Autodesk Inventor part; units mm, degrees
ref_plane "YZ Plane" through (0, 0, 0) normal (1, 0, 0) x (0, 1, 0)
ref_plane "XZ Plane" through (0, 0, 0) normal (0, 1, 0) x (-1, 0, 0)
ref_plane "XY Plane" through (0, 0, 0) normal (0, 0, 1) x (1, 0, 0)
sketch "Esquisse2" plane through (0, 0, 0) normal (0, 0, 1) x (1, 0, 0)
  line L0 (0, 0) -> (15, 0)
  line L1 (18, 3) -> (18, 33)
  line L2 (15, 36) -> (0, 36)
  line L3 (-3, 33) -> (-3, 3)
  line L4 (-3, 3) -> (0, 0)
  line L5 (0, 36) -> (-3, 33)
  line L6 (15, 36) -> (18, 33)
  line L7 (18, 3) -> (15, 0)
  line L8 (0, 36) -> (0, 0) construction
  line L9 (15, 0) -> (15, 36) construction
  line L10 (18, 33) -> (-3, 33) construction
  line L11 (18, 3) -> (-3, 3) construction
  dimension "d12" = 15
  dimension "d14" = 21
  dimension "d15" = 36
extrude "Extrusion1" add sketch "Esquisse2" along normal blind 24
sketch "Esquisse3" plane through (-3, 3, 0) normal (-1, 0, 0) x (0, 0, 1)
  line L0 (0, 0) -> (0, 30) construction
  line L1 (24, 30) -> (24, 0) construction
  line L2 (0, -3) -> (24, -3) construction
  line L3 (3, -3) -> (21, -3)
  line L4 (21, -3) -> (21, 2.6)
  line L5 (21, 2.6) -> (3, 2.6)
  line L6 (3, 2.6) -> (3, -3)
  line L7 (3, 2.6) -> (0, 2.6) construction
  line L8 (21, 2.6) -> (24, 2.6) construction
  dimension "d24" = 3
  dimension "d25" = 5.6
extrude "Extrusion2" cut sketch "Esquisse3" against normal through all
sketch "Esquisse4" plane through (0, 0, 0) normal (0, 0, -1) x (-1, 0, 0)
  line L0 (-15, 0) -> (0, 0) construction
  line L1 (0, 0) -> (3, 3) construction
  line L2 (0, 36) -> (-15, 36) construction
  circle A0 centre (-7.5, 3) radius 2.5
  line L3 (-15, 0) -> (-7.5, 3) construction
  line L4 (0, 0) -> (-7.5, 3) construction
  line L5 (-7.5, 3) -> (3, 3) construction
  circle A1 centre (-1.5, 3) radius 2.5
  circle A2 centre (-13.5, 3) radius 2.5
  circle A3 centre (-7.5, 3) radius 2.5
  dimension "d28" = 0.5
  dimension "d29" = 5
  dimension "d32" = 6
  dimension "d35" = 6
extrude "Extrusion3" cut sketch "Esquisse4" against normal through all
sketch "Esquisse5" plane through (0, 0, 0) normal (0, 0, -1) x (-1, 0, 0)
  circle A0 centre (-7.5, 3) radius 2.5 construction
  line L0 (3, 3) -> (3, 33) construction
  line L1 (0, 36) -> (-15, 36) construction
  line L2 (-7.5, 3) -> (-7.5, 36) construction
  circle A1 centre (-7.5, 27) radius 2.5
  line L3 (-7.5, 27) -> (3, 27) construction
  circle A2 centre (-1.5, 27) radius 2.5
  circle A3 centre (-13.5, 27) radius 2.5
  circle A4 centre (-7.5, 27) radius 2.5
  dimension "d40" = 5
  dimension "d41" = 24
  dimension "d44" = 6
  dimension "d47" = 6
extrude "Extrusion4" cut sketch "Esquisse5" against normal blind 3
sketch "Esquisse7" plane through (7.5, 27, 3) normal (0, 0, -1) x (-1, 0, 0)
  circle A0 centre (0, 0) radius 2.5
  circle A1 centre (0, 0) radius 2
  point P0 (7.5, -27)
  dimension "d54" = 4
extrude "Extrusion6" cut sketch "Esquisse7" against normal through all contours A1
sketch "Esquisse8" plane through (18, 3, 0) normal (1, 0, 0) x (0, 0, -1)
  line L0 (0, 30) -> (0, 0) construction
  line L1 (0, 26.5) -> (0, 21.5)
  line L2 (-24, 21.4697) -> (-24, 26.4697)
  line L3 (-24, 23.9697) -> (0, 24) construction
  line L4 (-21, 20.7349) -> (-3, 20.7349)
  line L5 (-3, 20.7349) -> (-3, 27.2349)
  line L6 (-3, 27.2349) -> (-21, 27.2349)
  line L7 (-21, 27.2349) -> (-21, 20.7349)
  line L8 (-21, 20.7349) -> (-3, 27.2349) construction
  line L9 (-3, 20.7349) -> (-21, 27.2349) construction
  line L10 (-21, 2.6) -> (-3, 2.6)
  line L11 (-12, 23.9849) -> (-12, 2.6) construction
  line L12 (-21, 2.7349) -> (-3, 2.7349)
  line L13 (-3, 2.7349) -> (-3, 9.2349)
  line L14 (-3, 9.2349) -> (-21, 9.2349)
  line L15 (-21, 9.2349) -> (-21, 2.7349)
  point P0 (0, -3)
  dimension "d57" = 6.5
  dimension "d58" = 18
  dimension "d74" = 18
extrude "Extrusion7" add sketch "Esquisse8" along normal blind 1.5
sketch "Esquisse9" plane through (19.5, 3, 0) normal (1, 0, 0) x (0, 0, -1)
  line L0 (-3, 20.7349) -> (-3, 27.2349) construction
  line L1 (-21, 27.2349) -> (-21, 20.7349) construction
  line L2 (-21, 23.9849) -> (-3, 23.9849) construction
  circle A0 centre (-12, 23.9849) radius 2.5
  line L3 (-15, 23.9849) -> (3, 23.9849) construction
  circle A1 centre (-6, 23.9849) radius 2.5
  line L4 (-27, 23.9849) -> (-9, 23.9849) construction
  circle A2 centre (-18, 23.9849) radius 2.5
  line L5 (-21, 23.9849) -> (-3, 23.9849) construction
  circle A3 centre (-12, 23.9849) radius 2.5
  line L6 (-21, 20.7349) -> (-3, 20.7349)
  line L7 (-12, 23.9849) -> (-12, 11.4292) construction
  circle A4 centre (-12, 5.9849) radius 2.5
  circle A5 centre (-6, 5.9849) radius 2.5
  circle A6 centre (-18, 5.9849) radius 2.5
  point P0 (0, -3)
  dimension "d61" = 5
  dimension "d64" = 6
  dimension "d67" = 6
  dimension "d81" = 18
extrude "Extrusion8" cut sketch "Esquisse9" against normal blind 3
sketch "Esquisse10" plane through (-3, 3, 0) normal (-1, 0, 0) x (0, 0, 1)
  line L0 (3, 27.2349) -> (21, 27.2349)
  line L1 (21, 27.2349) -> (21, 20.7349)
  line L2 (21, 20.7349) -> (3, 20.7349)
  line L3 (3, 20.7349) -> (3, 27.2349)
  line L4 (21, 9.2349) -> (21, 2.7349)
  line L5 (21, 2.7349) -> (3, 2.7349)
  line L6 (3, 2.7349) -> (3, 9.2349)
  line L7 (3, 9.2349) -> (21, 9.2349)
  point P0 (0, -3)
extrude "Extrusion9" add sketch "Esquisse10" along normal blind 1.5
sketch "Esquisse11" plane through (-4.5, 3, 0) normal (-1, 0, 0) x (0, 0, 1)
  circle A0 centre (6, 23.9849) radius 2.5
  circle A1 centre (12, 23.9849) radius 2.5
  circle A2 centre (18, 23.9849) radius 2.5
  circle A3 centre (18, 5.9849) radius 2.5
  circle A4 centre (12, 5.9849) radius 2.5
  circle A5 centre (6, 5.9849) radius 2.5
  point P0 (0, -3)
extrude "Extrusion10" cut sketch "Esquisse11" against normal blind 1.5
sketch "Esquisse12" plane through (-3, 3, 0) normal (-1, 0, 0) x (0, 0, 1)
  line L0 (21, 27.2349) -> (21, 20.7349)
  line L1 (21, 20.7349) -> (3, 20.7349)
  line L2 (3, 20.7349) -> (3, 27.2349)
  line L3 (3, 27.2349) -> (21, 27.2349)
  line L4 (21, 2.7349) -> (3, 2.7349)
  line L5 (3, 2.7349) -> (3, 9.2349)
  line L6 (3, 9.2349) -> (21, 9.2349)
  line L7 (21, 9.2349) -> (21, 2.7349)
  line L8 (21, 2.6) -> (21, 0)
  line L9 (21, 0) -> (24, 0)
  line L10 (24, 30) -> (24, 0)
  line L11 (0, 30) -> (24, 30)
  line L12 (0, 0) -> (0, 30)
  line L13 (0, 0) -> (3, 0)
  line L14 (3, 0) -> (3, 2.6)
  line L15 (3, 2.6) -> (21, 2.6)
  point P0 (0, -3)
sketch "Esquisse13" plane through (18, 3, 0) normal (1, 0, 0) x (0, 0, -1)
  line L0 (-21, 9.2349) -> (-3, 9.2349)
  line L1 (-3, 20.7349) -> (-18.5, 20.7349)
  line L2 (-18.5, 20.7349) -> (-18.5, 9.2349)
  line L3 (-18.5, 9.2349) -> (-3, 9.2349)
  line L4 (-3, 9.2349) -> (-3, 20.7349)
  point P0 (0, -3)
  dimension "d90" = 15.5
extrude "Extrusion11" cut sketch "Esquisse13" against normal blind 3
sketch "Esquisse14" plane through (18, 3, 0) normal (1, 0, 0) x (0, 0, -1)
  line L0 (-21, 20.7349) -> (-3, 20.7349)
  line L1 (-3, 9.2349) -> (-21, 9.2349)
  line L2 (-3, 20.7349) -> (-9, 20.7349)
  line L3 (-9, 20.7349) -> (-9, 9.2349)
  line L4 (-9, 9.2349) -> (-3, 9.2349)
  line L5 (-3, 9.2349) -> (-3, 20.7349)
  point P0 (0, -3)
  dimension "d93" = 6
extrude "Extrusion12" add sketch "Esquisse14" against normal blind 0.2
sketch "Esquisse16" plane through (-3, 3, 0) normal (-1, 0, 0) x (0, 0, 1)
  line L0 (3, 9.2349) -> (21, 9.2349) construction
  line L1 (3, 20.7349) -> (18.5, 20.7349)
  line L2 (18.5, 20.7349) -> (18.5, 9.2349)
  line L3 (18.5, 9.2349) -> (3, 9.2349)
  line L4 (3, 9.2349) -> (3, 20.7349)
  point P0 (0, -3)
  dimension "d96" = 15.5
extrude "Extrusion13" cut sketch "Esquisse16" against normal blind 3
sketch "Esquisse17" plane through (-3, 3, 0) normal (-1, 0, 0) x (0, 0, 1)
  line L0 (3, 20.7349) -> (9, 20.7349)
  line L1 (9, 20.7349) -> (9, 9.2197)
  line L2 (9, 9.2197) -> (3, 9.2197)
  line L3 (3, 9.2197) -> (3, 20.7349)
  line L4 (3, 9.2349) -> (3, 20.7349)
  point P0 (0, -3)
  dimension "d99" = 6
extrude "Extrusion14" add sketch "Esquisse17" against normal blind 0.2
fillet "Congé1" radius 1 9 edges at (18, 33, 12) (15, 36, 12) (0, 36, 12) (0, 0, 1.5) (0, 0, 22.5) (15, 0, 1.5) (18, 3, 1.5) (15, 0, 22.5) (18, 3, 22.5)
chamfer "Chanfrein1" distance 0.5 angle 45 2 edges at (-3, 17.9849, 18.5) (18, 17.9849, 18.5)
sketch "Esquisse18" plane through (0, 0, 24) normal (0, 0, 1) x (1, 0, 0)
  circle A0 centre (7.5, 27) radius 2
  circle A1 centre (1.5, 3) radius 2.5
  circle A2 centre (7.5, 3) radius 2.5
  circle A3 centre (13.5, 3) radius 2.5
  arc A4 (17.7071, 2.7071) -> (18, 3.4142) centre (17, 3.4142) ccw
  line L0 (18, 3.4142) -> (18, 32.5858)
  arc A5 (18, 32.5858) -> (17.7071, 33.2929) centre (17, 32.5858) ccw
  line L1 (17.7071, 33.2929) -> (15.2929, 35.7071)
  arc A6 (15.2929, 35.7071) -> (14.5858, 36) centre (14.5858, 35) ccw
  line L2 (14.5858, 36) -> (0.4142, 36)
  arc A7 (0.4142, 36) -> (-0.2929, 35.7071) centre (0.4142, 35) ccw
  line L3 (-0.2929, 35.7071) -> (-3, 33)
  line L4 (-3, 33) -> (-3, 3)
  line L5 (-3, 3) -> (-0.2929, 0.2929)
  arc A8 (-0.2929, 0.2929) -> (0.4142, 0) centre (0.4142, 1) ccw
  line L6 (0.4142, 0) -> (14.5858, 0)
  arc A9 (14.5858, 0) -> (15.2929, 0.2929) centre (14.5858, 1) ccw
  line L7 (15.2929, 0.2929) -> (17.7071, 2.7071)
  line L8 (19.5, 11.4849) -> (19.5, 6.4849)
  line L9 (19.5, 8.9849) -> (4.268, 8.9849) construction
  point P0 (0, 0)
properties part number "Motor"
Build history of the part. All positions in model axes, mm. A direction names the side the tool comes from. Coordinates: 2 decimals unless noted, no trailing zeros. Order: outer loops, then holes, each group sorted by start corner. A loop starts at its lowest first (then second) coordinate and runs counter-clockwise, first axis right, second up. Notation, with made-up numbers: (-28, 0.5) -> (7, 0.5) arc R29 cw to (7, 37.5) -> close; hole circle Ø4 at (-5.75, 44). An arc over 180 degrees is marked (long way). Answer in a Markdown table with one row per item. Add a question column.
Q1. Band-saw the part on D-D, the plane y = 4. Give the number of separate pieces and of enclosed holes in the cut face, then the cut area to 3 significant figures.
Q2. Band-saw the part on A-A, the plane x = 1.5. List the corners of the cut face in (y, z), then the cut area to 3 significant figures.
Q3. Band-saw the part on C-C, the plane x = 7.5. List the corners of the cut face in (y, z), then the cut area to 3 significant figures.
Q4. Mould opens along Y. For faces 1 (the face through (-4, 27, 3)), 2 (the face through (-1, 18, 3)), 3 (the face through (7, 0, 22)) say: +Y half, -Y half, draft (parallel to the pull), parting line (faces both ways), or undercut.
Q5. Which spindle directions (+Z, -Z, +X, -X, +Y, -Y) get a long thin tool onto all of the face, cutting with end or side? Do faces 4 (the face through (-3.76, 28.675, 16.157)), 5 (the face through (16.5, 27, 12)), 6 (the face through (19, 9, 21)), 7 (the face through (17.8, 18, 6)). Say none if no direction does.
Q6. Drop flat-ended pins along their axis: pin 1 (5.5 mm diameter, centred on y = 26, z = 19, fed in from +X); pin 2 (2 mm diameter, centred on x = 17, z = 10, fed in from -Y); pin 3 (3.5 mm diameter, centred on x = -3, z = 13, fed in from +Y); pin 4 (1.2 mm diameter, centred on x = -4, y = 8.5, fed in from +Z). Give the stop position or say it passes through.
Q7. Band-saw the part on B-B, the plane z = 22. List the corners of the cut face in (x, y).
Q8. Wall check: line 1 along Y through (x, z) = (-3.65, 12); line 2 along Z through (x, y) = (18.75, 9); line 3 along Y through (x, z) = (7.5, 1.15). Give the ranges that are in metal, low to high. Write a range as [from, to].
Answers follow:
| question | item | result |
|---|---|---|
| 1 | separate pieces | 8 |
| 1 | enclosed holes | 0 |
| 1 | area | 43.5 mm^2 |
| 2 | outline | (0, 0) -> (0.5, 0) -> (0.5, 3) -> (0, 3) -> close; (0, 21) -> (0.5, 21) -> (0.5, 24) -> (0, 24) -> close; (5.5, 0) -> (24.5, 0) -> (24.5, 3) -> (29.5, 3) -> (29.5, 0) -> (36, 0) -> (36, 24) -> (5.5, 24) -> (5.5, 21) -> (5.6, 21) -> (5.6, 3) -> (5.5, 3) -> close |
| 2 | area | 718 mm^2 |
| 3 | outline | (0, 0) -> (0.5, 0) -> (0.5, 3) -> (0, 3) -> close; (0, 21) -> (0.5, 21) -> (0.5, 24) -> (0, 24) -> close; (5.5, 0) -> (24.5, 0) -> (24.5, 3) -> (25, 3) -> (25, 24) -> (5.5, 24) -> (5.5, 21) -> (5.6, 21) -> (5.6, 3) -> (5.5, 3) -> close; (29, 3) -> (29.5, 3) -> (29.5, 0) -> (36, 0) -> (36, 24) -> (29, 24) -> close |
| 3 | area | 634 mm^2 |
| 4 | face 1 | draft |
| 4 | face 2 | undercut |
| 4 | face 3 | -Y half |
| 5 | face 4 | -X |
| 5 | face 5 | +X |
| 5 | face 6 | +Z, +X, +Y, -Y |
| 5 | face 7 | none |
| 6 | pin 1 | x = 19.5 |
| 6 | pin 2 | y = 5.6 |
| 6 | pin 3 | y = 34.75 |
| 6 | pin 4 | z = 21 |
| 7 | outline | (-3, 3) -> (-0.29, 0.29) arc R1 ccw to (0.41, 0) -> (14.59, 0) arc R1 ccw to (15.29, 0.29) -> (17.71, 2.71) arc R1 ccw to (18, 3.41) -> (18, 32.59) arc R1 ccw to (17.71, 33.29) -> (15.29, 35.71) arc R1 ccw to (14.59, 36) -> (0.41, 36) arc R1 ccw to (-0.29, 35.71) -> (-3, 33) -> close; hole circle Ø5 at (1.5, 3); hole circle Ø5 at (7.5, 3); hole circle Ø4 at (7.5, 27); hole circle Ø5 at (13.5, 3) |
| 8 | line 1 | [5.73, 6.48], [11.48, 12.23], [23.73, 24.48], [29.48, 30.23] |
| 8 | line 2 | [3, 3.5], [8.5, 9.5], [14.5, 15.5], [20.5, 21] |
| 8 | line 3 | [0, 0.5], [5.5, 24.5], [29.5, 36] |
